The listing builds one solid part. Answer for the finished solid, in the listing's coordinates (mm). Give positions to 0.01 mm unless a question says otherwise; leave off trailing zeros. Write each loop counter-clockwise with the first axis right and the second up, starting at its lowest first coordinate (ties: lowest second). Pieces come first, ordered by that corner, then holes. Notation, with made-up numbers: M 81,57 L 132,57 A22 cw 132,79 Z; hole C 57.25,39.25 d7. An arc over 180 degrees is marked long. Answer as a JSON object with one key per item and string values.
```python
from build123d import *

# Parameters (mm, degrees)
SKETCH_1_W          = 18.46
SKETCH_1_H          = 19.3
EXTRUDE_1_DEPTH     = 1
SKETCH_2_W          = 9.46
SKETCH_2_H          = 4.5
CUT_EXTRUDE_1_DEPTH = 14.390870024
FILLET_1_R          = 1.56
CUT_EXTRUDE_2_DEPTH = 14.390870024
FILLET_7_R          = 0.55


with BuildPart() as part:
    # 草图1 → 凸台-拉伸1 (new body)
    with BuildSketch(Plane(origin=(0, 0, 0), x_dir=(1, 0, 0), z_dir=(0, 1, 0))):
        Rectangle(SKETCH_1_W, SKETCH_1_H)
    extrude(amount=EXTRUDE_1_DEPTH)

    # 草图2 → 切除-拉伸1 (cut, through all)
    with BuildSketch(Plane.XZ):
        with Locations((0, -7.4)):
            Rectangle(SKETCH_2_W, SKETCH_2_H)
    extrude(amount=-CUT_EXTRUDE_1_DEPTH, mode=Mode.SUBTRACT)

    # 圆角1
    fillet_1_edges = [part.edges().sort_by_distance(p)[0] for p in [
        (4.73, 0.5, -5.15),
        (-4.73, 0.5, -5.15),
    ]]
    fillet(fillet_1_edges, radius=FILLET_1_R)

    # 草图3 → 切除-拉伸2 (cut, through all)
    with BuildSketch(Plane(origin=(0, 1, 0), x_dir=(1, 0, 0), z_dir=(0, 1, 0))):
        Polygon((1, 3.1), (3.1, 3.1), (3.1, -3.1), (-3.1, -3.1), (-3.1, 3.1), (-1, 3.1), (-1, 2), (-2, 2), (-2, -2), (2, -2), (2, 2), (1, 2), align=None)
    extrude(amount=-CUT_EXTRUDE_2_DEPTH, mode=Mode.SUBTRACT)

    # 圆角7
    fillet_7_edges = [part.edges().sort_by_distance(p)[0] for p in [
        (-1, 0.5, -2),
        (1, 0.5, -2),
        (-3.1, 0.5, 3.1),
        (-1, 0.5, -3.1),
        (-3.1, 0.5, -3.1),
        (1, 0.5, -3.1),
        (3.1, 0.5, -3.1),
        (3.1, 0.5, 3.1),
    ]]
    fillet(fillet_7_edges, radius=FILLET_7_R - 0.0001)  # a hair under: the kernel refuses the full size


solid = part.part
```
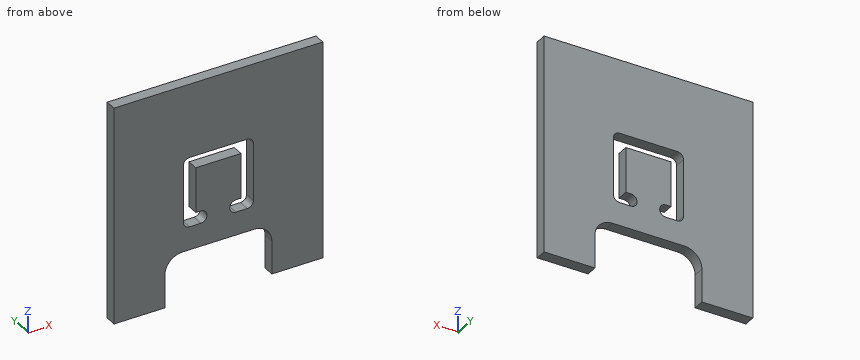
1. Consider line 1 along X through (y, z) = (0.1, -1.75); line 2 along Z through (x, y) = (-2.5, 0.8); line 3 along Z through (x, y) = (0, 0.5). Determine where each line is inside the solid, lowest interval first.
Verdict:
{"line 1": "x = -9.23 to -3.1, -2 to 2, 3.1 to 9.23", "line 2": "z = -5.15 to -3.1, 3.1 to 9.65", "line 3": "z = -5.15 to 2, 3.1 to 9.65"}
2. A flat-ended cylindrical pin translates along its axis: pin 1 (0.5 mm diameter, centred on x = -1, y = 0.5, fed in from -Z). Find the tip coordinate at first contact, or state that the pin passes through.
Verdict:
{"pin 1": "stops at z = -5.15"}
3. A cutting plane is placed at C-C, the plane z = -7.5. Give the vertices of the cut face in (x, y).
Verdict:
{"outline": "M -9.23,0 L -4.73,0 L -4.73,1 L -9.23,1 Z; M 4.73,0 L 9.23,0 L 9.23,1 L 4.73,1 Z"}
4. A cutting plane is placed at A-A, the plane z = 2.25. Give the vertices of the cut face in (x, y).
Verdict:
{"outline": "M -9.23,0 L -3.1,0 L -3.1,1 L -9.23,1 Z; M 3.1,0 L 9.23,0 L 9.23,1 L 3.1,1 Z"}
5. A cutting plane is placed at D-D, the plane x = 3.5. Give the vertices of the cut face in (y, z), plus the area to 3 significant figures.
Verdict:
{"outline": "M 0,-5.19 L 1,-5.19 L 1,9.65 L 0,9.65 Z", "area": "14.8 mm2"}
